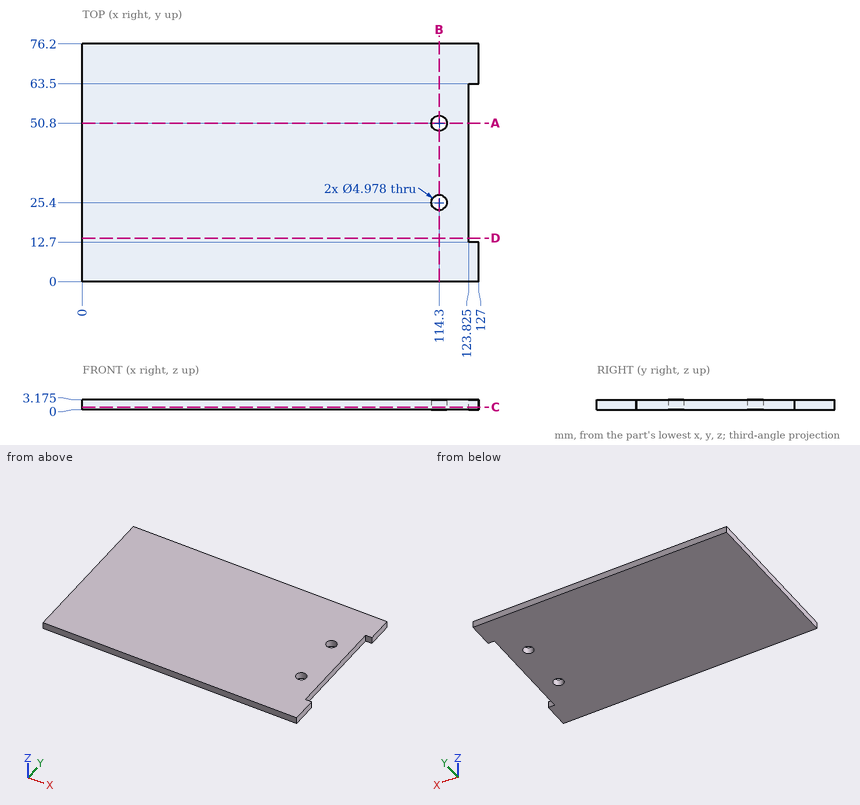
Verification items for this drawing (mm, ordinates from the low corner). Coordinates: 2 decimals unless noted, no trailing zeros. Write each loop counter-clockwise with the first axis right and the second up, starting at its lowest first coordinate (ties: lowest second). Pieces come first, ordered by that corner, then holes. Notation, with made-up numbers: M 56,21 L 94,21 A20 cw 94,27 Z; hole C -36,82 d3. An arc over 180 degrees is marked long. Use one line per item in the form item = value. Start each with the question number.
1) Go/stop test with a flat-tipped pin: pin 1 Ø1 at (y, z) = (36.5, 1) entering from +X (3 decimals). Record where the tip stops, or that it passes through.
2) Section check D-D on y = 14. Enter the section's corners in (x, z) (1 decimal), and give its area (3 significant figures).
3) Section check A-A on y = 50.8. Enter the section's corners in (x, z) (1 decimal).
4) Section check C-C on z = 0.85. Enter the section's corners in (x, y) (1 decimal).
5) Section check B-B on x = 114.3. Enter the section's corners in (y, z) (1 decimal), and give its area (3 significant figures).
6) Thickness scan on probe 1 along Y at (x, z) = (114.3, 2.4); probe 2 along X at (y, z) = (60, 2.1) (1 decimal); probe 3 along X at (y, z) = (26, 2.25) (1 decimal). Record the ranges inside material, lowest first. Write a range as from..to.
Responses:
q1.pin_1 = 123.825
q2.outline = M 0,0 L 123.8,0 L 123.8,3.2 L 0,3.2 Z
q2.area = 393 mm2
q3.outline = M 0,0 L 111.8,0 L 111.8,3.2 L 0,3.2 Z; M 116.8,0 L 123.8,0 L 123.8,3.2 L 116.8,3.2 Z
q4.outline = M 0,0 L 127,0 L 127,12.7 L 123.8,12.7 L 123.8,63.5 L 127,63.5 L 127,76.2 L 0,76.2 Z; hole C 114.3,25.4 d5; hole C 114.3,50.8 d5
q5.outline = M 0,0 L 22.9,0 L 22.9,3.2 L 0,3.2 Z; M 27.9,0 L 48.3,0 L 48.3,3.2 L 27.9,3.2 Z; M 53.3,0 L 76.2,0 L 76.2,3.2 L 53.3,3.2 Z
q5.area = 210 mm2
q6.probe_1 = 0..22.91, 27.89..48.31, 53.29..76.2
q6.probe_2 = 0..123.8
q6.probe_3 = 0..111.9, 116.7..123.8
